Could you check a few things on this model? Use its own coordinates, in mm. A direction names the side the tool comes from. Give positions to 0.01 mm unless a question says otherwise; leave off trailing zeros. Write each loop counter-clockwise with the first axis right and the second up, starting at its lowest first coordinate (ties: lowest second). Pieces come first, ordered by that corner, then holes. Notation, with made-up numbers: (75.5, 21.5) - (105.5, 21.5) arc R19 cw to (105.5, 57.5) - close; hole circle Ø9 at (78.25, 78). An arc over 180 degrees is marked (long way). Answer in a Markdown table with one row per item.
from build123d import *

# Parameters (mm, degrees)
BOSS_EXTRUDE1_DEPTH      = 1
BOSS_EXTRUDE1_DEPTH_BACK = 2
SKETCH1_R                = 3.5
SKETCH1_R_2              = 1.65
SKETCH2_R                = 4.75
BOSS_EXTRUDE2_DEPTH      = 2.5
SKETCH3_R                = 4.125
CUT_EXTRUDE1_DEPTH       = 2.1
FILLET1_R                = 0.5
SKETCH4_R                = 1.65
CUT_EXTRUDE2_DEPTH       = 10
SKETCH5_W                = 15.11331488
SKETCH5_H                = 2
CUT_EXTRUDE3_DEPTH       = 3
FILLET2_R                = 2


with BuildPart() as part:
    # Sketch1 → Boss-Extrude1 (new, two sides: drawn at the far end of the back side and taken through both)
    with BuildSketch(Plane.XY.offset(-BOSS_EXTRUDE1_DEPTH_BACK)):
        Circle(SKETCH1_R)
        Circle(SKETCH1_R_2, mode=Mode.SUBTRACT)
    extrude(amount=BOSS_EXTRUDE1_DEPTH + BOSS_EXTRUDE1_DEPTH_BACK)

    # Sketch2 → Boss-Extrude2 (add)
    with BuildSketch(Plane.XY.offset(1)):
        Circle(SKETCH2_R)
    extrude(amount=BOSS_EXTRUDE2_DEPTH)

    # Sketch3 → Cut-Extrude1 (cut)
    with BuildSketch(Plane.XY.offset(3.5)):
        Circle(SKETCH3_R)
    extrude(amount=-CUT_EXTRUDE1_DEPTH, mode=Mode.SUBTRACT)

    # Fillet1
    fillet1_edges = [part.edges().sort_by_distance(p)[0] for p in [
        (-4.125, 0, 3.5),
    ]]
    fillet(fillet1_edges, radius=FILLET1_R)

    # Sketch4 → Cut-Extrude2 (cut)
    with BuildSketch(Plane(origin=(0, 0, -2), x_dir=(-1, 0, 0), z_dir=(0, 0, -1))):
        with Locations(Location((0, 0, 0), (0, 0, 180))):
            Circle(SKETCH4_R)
    extrude(amount=-CUT_EXTRUDE2_DEPTH, mode=Mode.SUBTRACT)

    # Sketch5 → Cut-Extrude3 (cut)
    with BuildSketch(Plane.XY.offset(1.4)):
        Rectangle(SKETCH5_W, SKETCH5_H)
    extrude(amount=CUT_EXTRUDE3_DEPTH, mode=Mode.SUBTRACT)

    # Fillet2
    # the kernel refuses this fillet: 2 mm, written as the material it adds along each edge
    with BuildSketch(Plane(origin=(0, 0, 1), x_dir=(1, 0, 0), z_dir=(0, -1, 0))) as fillet2_piece_1:
        with BuildLine():
            CenterArc((5.5, -1.854049622), FILLET2_R, 112.024312837, 67.975687163)
            Line((4.75, 0), (4.735, 0.037080992))
            ThreePointArc((4.735, 0.037080992), (4.125, 0.04), (3.5, 0.04))
            Line((3.5, 0.04), (3.46, 0))
            Line((3.46, 0), (3.46, -1.854049622))
            Line((3.46, -1.854049622), (3.5, -1.854049622))
        make_face()
    revolve(axis=Axis((0, 0, 1), (0, 0, 1)))


solid = part.part
1) Imagine slicing it at D-D (z = -1.3). List the corners of the cut face in (x, y) for me.
Check values:
| item | result |
|---|---|
| outline | circle Ø7 at (0, 0); hole circle Ø3.3 at (0, 0) |
2) Imagine slicing it at C-C (y = 0). List the corners of the cut face in (x, z) for me, then the cut area to 3 significant figures.
Check values:
| item | result |
|---|---|
| outline | (-4.75, 1) arc R2 cw to (-3.5, -0.85) - (-3.5, -2) - (-1.65, -2) - (-1.65, 1.4) - (-4.75, 1.4) - close; (1.65, -2) - (3.5, -2) - (3.5, -0.85) arc R2 cw to (4.75, 1) - (4.75, 1.4) - (1.65, 1.4) - close |
| area | 14.9 mm2 |
3) On a 3-axis mill with a long thin cutter (end or side, diameter ignored), from which of +Z, -Z, +X, -X, +Y, -Y can I reach the whole of each face in a straight line? I mean faces 4 (the face through (-0.077, -4.124, 2.211)), 5 (the face through (3.233, -1.341, -1.435)). Say none if no direction works.
Check values:
| item | result |
|---|---|
| face 4 | +Z |
| face 5 | -Z |
4) We'd pull the mould along Y, two halves only. Please class faces 1 (the face through (4.388, -1.819, 2.232)), 2 (the face through (-1.216, -1.115, -0.324)), 3 (the face through (1, -2, -2)): +Y half, -Y half, draft (parallel to the pull), parting line (faces both ways), or undercut.
Check values:
| item | result |
|---|---|
| face 1 | parting line |
| face 2 | undercut |
| face 3 | draft |
5) Imagine slicing it at A-A (x = 0). List the corners of the cut face in (y, z) for me (3 decimals), then the cut area to 3 significant figures.
Check values:
| item | result |
|---|---|
| outline | (-4.75, 1) arc R2 cw to (-3.5, -0.854) - (-3.5, -2) - (-1.65, -2) - (-1.65, 1.4) - (-4.125, 1.4) - (-4.125, 3) arc R0.5 ccw to (-4.625, 3.5) - (-4.75, 3.5) - close; (1.65, -2) - (3.5, -2) - (3.5, -0.854) arc R2 cw to (4.75, 1) - (4.75, 3.5) - (4.625, 3.5) arc R0.5 ccw to (4.125, 3) - (4.125, 1.4) - (1.65, 1.4) - close |
| area | 17.4 mm2 |
6) If I drill on line 1 (Y direction, x = 0, z = 0.6); line 2 (Z direction, x = 0.75, y = -1.75); line 3 (X direction, y = -3.75, z = 1.95), over which ranges is the centre line in solid material (lowest first)?
Check values:
| item | result |
|---|---|
| line 1 | y = -4.13 to -1.65, 1.65 to 4.13 |
| line 2 | z = -2 to 1.4 |
| line 3 | x = -2.92 to -1.72, 1.72 to 2.92 |
7) Imagine slicing it at B-B (z = 2.75). List the corners of the cut face in (x, y) for me (3 decimals).
Check values:
| item | result |
|---|---|
| outline | (-4.644, -1) arc R4.75 ccw to (4.644, -1) - (4.002, -1) arc R4.125 cw to (-4.002, -1) - close; (-4.644, 1) - (-4.002, 1) arc R4.125 cw to (4.002, 1) - (4.644, 1) arc R4.75 ccw to start |
8) Will these pins go through, and if not, where does the flat tip stop? P1, Ø4, axis at x = 1.5, y = -0.5, coming from the +Z side; P2, Ø1.5, axis at y = 0.5, z = 2.5, coming from the -X side; P3, Ø0.7, axis at x = 4.5, z = 2, coming from the +Y side.
Check values:
| item | result |
|---|---|
| P1 | stops at z = 1.4 |
| P2 | stops at x = -4.64 |
| P3 | stops at y = 2.31 |
